Here's how the part is built. I have some questions about the finished solid (model axes, mm). Round coordinates to 2 decimals unless told otherwise and drop trailing zeros. Write each loop counter-clockwise with the first axis right and the second up, starting at its lowest first coordinate (ties: lowest second). Pieces come first, ordered by that corner, then holes. Notation, with made-up numbers: (55.5, 84) -> (104.5, 84) arc R18 cw to (104.5, 99) -> close; hole circle Ø11 at (-12.5, 25.5). An arc over 180 degrees is marked (long way). Answer in a Markdown table with one row per item.
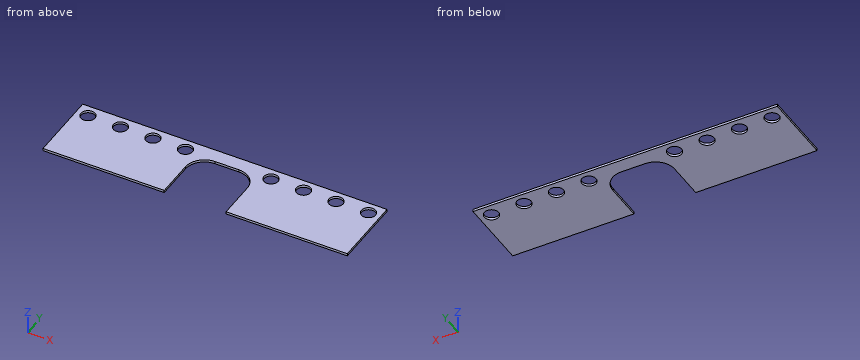
Autodesk Inventor part; units mm, degrees
ref_plane "YZ Plane" through (0, 0, 0) normal (1, 0, 0) x (0, 1, 0)
ref_plane "XZ Plane" through (0, 0, 0) normal (0, 1, 0) x (-1, 0, 0)
ref_plane "XY Plane" through (0, 0, 0) normal (0, 0, 1) x (1, 0, 0)
sketch "Sketch1" plane through (0, 0, 0) normal (0, 0, 1) x (1, 0, 0)
  line L0 (812.8, 0) -> (812.8, 190.5)
  line L1 (812.8, 190.5) -> (0, 190.5)
  line L2 (0, 190.5) -> (0, 0)
  circle A0 centre (781.05, 158.75) radius 19.05
  circle A1 centre (520.7, 158.75) radius 19.05
  circle A2 centre (292.1, 158.75) radius 19.05
  circle A3 centre (31.75, 158.75) radius 19.05
  circle A4 centre (694.2667, 158.75) radius 19.05
  circle A5 centre (205.3167, 158.75) radius 19.05
  circle A6 centre (607.4833, 158.75) radius 19.05
  circle A7 centre (118.5333, 158.75) radius 19.05
  line L3 (488.95, 0) -> (488.95, 101.6)
  line L4 (488.95, 152.4) -> (438.15, 152.4) construction
  line L5 (323.85, 152.4) -> (323.85, 101.6) construction
  line L6 (0, 0) -> (323.85, 0)
  line L7 (488.95, 0) -> (812.8, 0)
  arc A8 (374.65, 152.4) -> (323.85, 101.6) centre (374.65, 101.6) ccw
  arc A9 (488.95, 101.6) -> (438.15, 152.4) centre (438.15, 101.6) ccw
  line L8 (374.65, 152.4) -> (323.85, 152.4) construction
  line L9 (323.85, 101.6) -> (323.85, 0)
  line L10 (438.15, 152.4) -> (374.65, 152.4)
  line L11 (488.95, 101.6) -> (488.95, 152.4) construction
  dimension "d0" = 190.5
  dimension "d1" = 812.8
  dimension "d13" = 38.1
  dimension "d14" = 38.1
  dimension "d15" = 228.6
  dimension "d16" = 260.35
  dimension "d17" = 86.7833
  dimension "d18" = 86.7833
  dimension "d21" = 31.75
  dimension "d22" = 31.75
  dimension "d23" = 31.75
  dimension "d24" = 86.7833
  dimension "d25" = 86.7833
  dimension "d26" = 165.1
  dimension "d28" = 323.85
  dimension "d29" = 152.4
  dimension "d30" = 50.8
extrude "Extrusion1" add sketch "Sketch1" along normal blind 6.35
equation "\"d14\" = d13"
equation "\"d16\" = 0.5 * d1 - 0.5 * d15 - d23"
equation "\"d17\" = 0.333333 * d16"
equation "\"d18\" = d17"
equation "\"d23\" = d22"
equation "\"d24\" = d17"
equation "\"d25\" = d18"
equation "\"d28\" = -0.5 * d26 + 0.5 * d1"
properties part number "manipulator back pannel 2"
1) I want a section at A-A, the plane y = 27.5. List the corners of the cut face in (x, z) for me, and give its area (3 significant figures).
Response:
| item | result |
|---|---|
| outline | (0, 0) -> (323.85, 0) -> (323.85, 6.35) -> (0, 6.35) -> close; (488.95, 0) -> (812.8, 0) -> (812.8, 6.35) -> (488.95, 6.35) -> close |
| area | 4,110 mm^2 |
2) I want a section at B-B, the plane x = 781.05. List the corners of the cut face in (y, z) for me.
Response:
| item | result |
|---|---|
| outline | (0, 0) -> (139.7, 0) -> (139.7, 6.35) -> (0, 6.35) -> close; (177.8, 0) -> (190.5, 0) -> (190.5, 6.35) -> (177.8, 6.35) -> close |
3) I want a section at C-C, the plane z = 5.25. Count the separate pieces of the cut face and the enclosed holes in it, and give its area (3 significant figures).
Response:
| item | result |
|---|---|
| separate pieces | 1 |
| enclosed holes | 8 |
| area | 122,000 mm^2 |
4) I need wall thicknesses on line 1 (Y direction, x = 520.7, z = 3.75); line 2 (X direction, y = 70.5, z = 1.25); line 3 (X direction, y = 103, z = 3.25). Which ranges of each line are inside material? Lowest first, please. Write a range as [from, to].
Response:
| item | result |
|---|---|
| line 1 | y = [0, 139.7], [177.8, 190.5] |
| line 2 | x = [0, 323.85], [488.95, 812.8] |
| line 3 | x = [0, 323.87], [488.93, 812.8] |
